The drawing under review shows one solid part. Ordinate dimensions are in mm from its lowest x, y, z. A direction names the side the tool comes from. Coordinates: 2 decimals unless noted, no trailing zeros. Write each loop counter-clockwise with the first axis right and the second up, starting at its lowest first coordinate (ties: lowest second). Pieces come first, ordered by that corner, then holes. Notation, with made-up numbers: (89, 13) -> (123, 13) arc R10 ccw to (123, 26) -> close; hole circle Ø4 at (36.25, -3). An arc over 180 degrees is marked (long way). One line per item, written item: value. Start each with the question number.
1) Machinability: for the marked faces 1 and 2, which of the approach directions +Z, -Z, +X, -X, +Y, -Y give a long, thin tool a straight path to every point of the face, cutting with its end or side? Answer none if there is none.
2) For probe 1 along Z at (x, y) = (8, 4.75); probe 2 along Z at (x, y) = (4, 5); probe 3 along Z at (x, y) = (6.75, 1.25), list the stretches that pass through material, from the lowest coordinate up. Write a range as from..to.
3) Add section C-C (z = 3.75). State the section outline as (x, y) points (3 decimals), and give its area (4 significant figures).
4) Add section B-B (y = 13.25). State the section outline as (x, z) points (3 decimals).
5) Add section A-A (y = 9). State the section outline as (x, z) points (3 decimals), and give its area (3 significant figures).
6) For pin 1 Ø4 at (x, y) = (9.5, 2) entering from -Z; pin 2 Ø2 at (y, z) = (3.5, 3) entering from +X; pin 3 Ø4 at (x, z) = (7.925, 3.325) entering from -Y (3 decimals), all flat-tipped, find the tip position at first contact; note any pin that passes through.
7) Add section D-D (z = 16.5). State the section outline as (x, y) points (3 decimals).
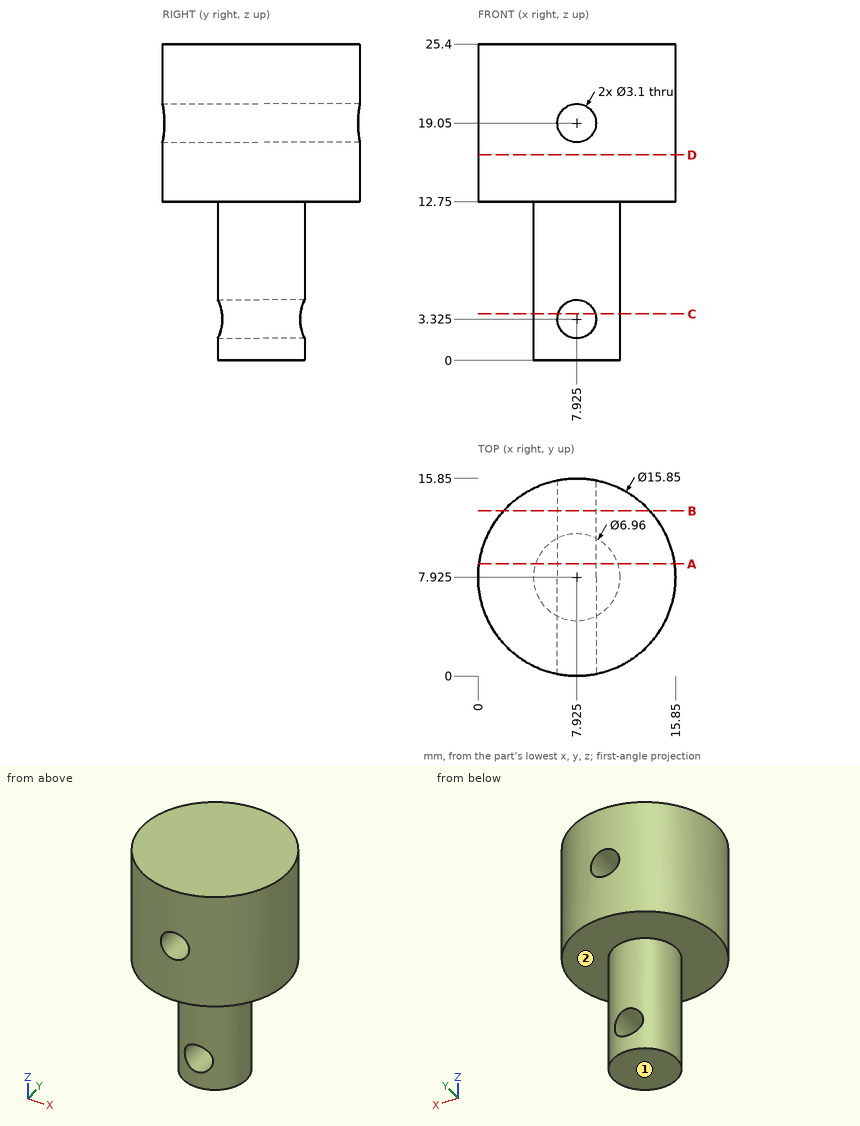
Numbers:
1. face 1: -Z, +X, -X, +Y, -Y
1. face 2: -Z
2. probe 1: 0..1.78, 4.87..17.5, 20.6..25.4
2. probe 2: 12.75..25.4
2. probe 3: 12.75..18.04, 20.06..25.4
3. outline: (6.434, 4.78) -> (6.434, 11.07) arc R3.48 ccw to start; (9.416, 4.78) arc R3.48 ccw to (9.416, 11.07) -> close
3. area: 17.95 mm²
4. outline: (2.056, 12.75) -> (13.794, 12.75) -> (13.794, 25.4) -> (2.056, 25.4) -> close; hole circle Ø3.1 at (7.925, 19.05)
5. outline: (0.073, 12.75) -> (4.615, 12.75) -> (4.615, 0) -> (11.235, 0) -> (11.235, 12.75) -> (15.777, 12.75) -> (15.777, 25.4) -> (0.073, 25.4) -> close; hole circle Ø3.1 at (7.925, 3.325); hole circle Ø3.1 at (7.925, 19.05)
5. area: 268 mm²
6. pin 1: z = 12.75
6. pin 2: through
6. pin 3: y = 4.445
7. outline: circle Ø15.85 at (7.925, 7.925)
